Could you check a few things on this drawing? It's one solid part, dimensions in mm from its lowest x, y, z. Coordinates: 2 decimals unless noted, no trailing zeros. Order: outer loops, then holes, each group sorted by start corner. A loop starts at its lowest first (then second) coordinate and runs counter-clockwise, first axis right, second up. Notation, with made-up numbers: M 43,-32 L 88,-32 A28 ccw 88,-4 Z; hole C 54,-12 d11. An arc over 180 degrees is marked long. Answer as CSV lines item,"result". Start each with the question number.
1. If we section it at D-D (x = 49): List the corners of the cut face in (y, z) for me, plus the area to 3 significant figures.
2. If we section it at A-A (y = 33): List the corners of the cut face in (x, z) for me.
3. Will these pins go through, and if not, where does the flat tip stop? pin 1 (2 mm diameter, centred on x = 39, z = 5, fed in from -Y); pin 2 (2 mm diameter, centred on y = 52.5, z = 11, fed in from +X); pin 3 (1 mm diameter, centred on x = 41.5, z = 10, fed in from -Y).
4. If we section it at B-B (z = 7.5): List the corners of the cut face in (x, y) for me.
5. If we section it at C-C (x = 10.5): List the corners of the cut face in (y, z) for me.
6. If we mould it in two halves opening along Y, with no side actions, what happens to the marked faces 1, 2 and 3? For each: released by +Y, released by -Y, zero draft, split by the parting line, or undercut.
7. I need wall thicknesses on line 1 along Z through (x, y) = (45, 3.5); line 2 along Y through (x, z) = (33, 3.5); line 3 along X through (y, z) = (30, 9.5). Which ranges of each line are inside material? Lowest first, please. Write a range as from..to.
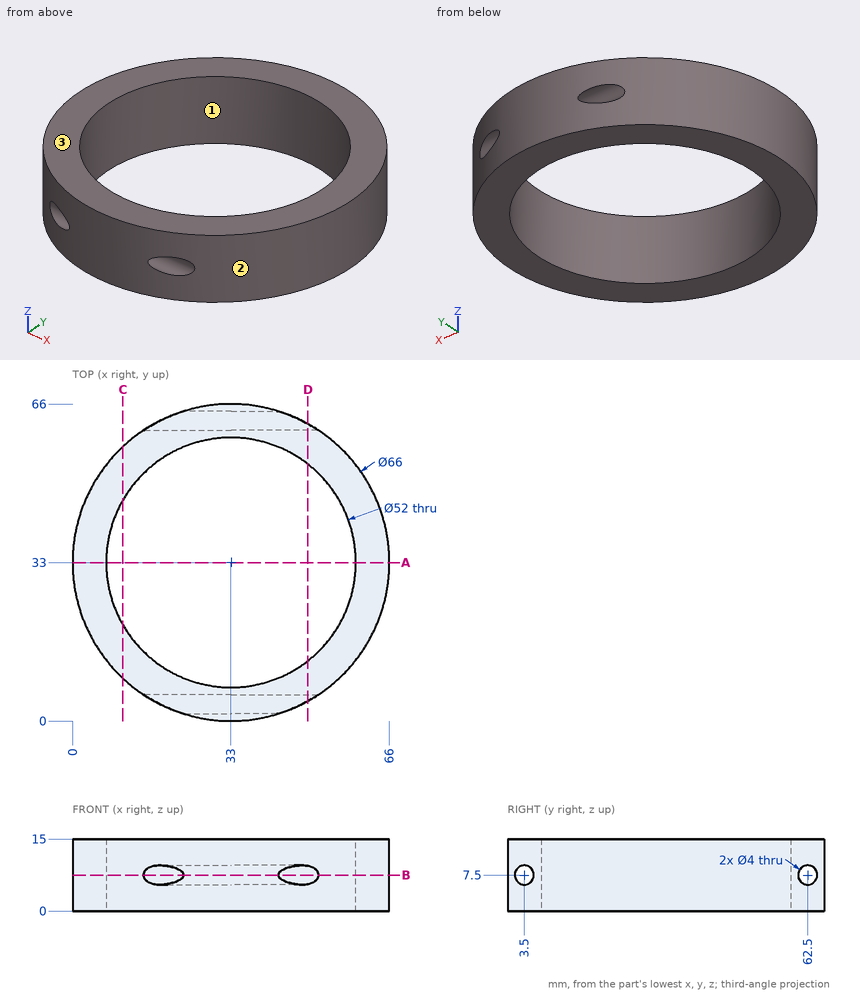
Solved:
1,outline,"M 4.14,0 L 12.51,0 L 12.51,15 L 4.14,15 L 4.14,9.4 A2 cw 4.14,5.6 Z; M 53.49,0 L 61.86,0 L 61.86,5.6 A2 cw 61.86,9.4 L 61.86,15 L 53.49,15 Z"
1,area,"243 mm²"
2,outline,"M 0,0 L 7,0 L 7,15 L 0,15 Z; M 59,0 L 66,0 L 66,15 L 59,15 Z"
3,pin 1,"y = 0.38"
3,pin 2,"x = 60.33"
3,pin 3,"y = 0.98"
4,outline,"M 14.76,5.5 L 51.24,5.5 A33 ccw 51.24,60.5 L 14.76,60.5 A33 ccw Z; M 23.16,1.5 A33 ccw 42.84,1.5 Z; M 23.16,64.5 L 42.84,64.5 A33 ccw Z; hole C 33,33 d52"
5,outline,"M 8.86,0 L 19.97,0 L 19.97,15 L 8.86,15 Z; M 46.03,0 L 57.14,0 L 57.14,15 L 46.03,15 Z"
6,face 1,"undercut"
6,face 2,"split by the parting line"
6,face 3,"zero draft"
7,line 1,"0..5.5, 9.5..15"
7,line 2,"0..7, 59..66"
7,line 3,"0.14..7.17, 58.83..65.86"
